Here's how the part is built. I have some questions about the finished solid (model axes, mm). Face numbers are marked on the shaded views. A direction names the side the tool comes from. Round coordinates to 2 decimals unless told otherwise and drop trailing zeros. Write each loop counter-clockwise with the first axis right and the second up, starting at its lowest first coordinate (ties: lowest second). Pieces come first, ordered by that corner, then holes. Notation, with made-up numbers: (2.25, -24.5) -> (18.25, -24.5) arc R14 ccw to (18.25, -5.5) -> close; hole circle Ø9 at (61.5, 24). An arc over 180 degrees is marked (long way). Put each result on its own line as item: value. Start each with the question number.
1) I want a section at B-B, the plane x = 23.5. List the corners of the cut face in (y, z) for me, then the cut area to 3 significant figures.
2) I want a section at C-C, the plane x = 7.5. List the corners of the cut face in (y, z) for me.
3) If I drill on line 1 along Z through (x, y) = (-34.5, -18.25); line 2 along Z through (x, y) = (38, -14); line 3 along Z through (x, y) = (35, -17), over which ranges is the centre line in solid material (lowest first)? Write a range as [from, to].
4) Will these pins go through, and if not, where does the flat tip stop? P1, Ø2, axis at y = -6, z = 25.5, coming from the -X side; P2, Ø1, axis at y = -19.5, z = 26.5, coming from the +X side; P3, Ø1, axis at x = 11, y = -19.5, coming from the +Z side.
5) Which directions (+Z, -Z, +X, -X, +Y, -Y) give clear straight access to the entire face, cutting with the end or side of a thin tool? Please do the marked faces 1 and 2.
6) I want a section at D-D, the plane z = 22.5. List the corners of the cut face in (x, y) for me, then the cut area to 3 significant figures.
7) I want a section at A-A, the plane y = -13.75. List the corners of the cut face in (x, z) for me.
from build123d import *

# Parameters (mm, degrees)
F1_DEPTH = 25


with BuildPart() as f1:
    # F0 (on Front) → F1 (new body)
    with BuildSketch(Plane.XZ):
        with BuildLine():
            Line((45.7854280798, 23.3870821038), (-39.147809339, 23.3870821038))
            ThreePointArc((-39.147809339, 23.3870821038), (-39.9978092392, 22.5370822037), (-39.147809339, 21.6870823036))
            Line((-39.147809339, 21.6870823036), (45.7854280798, 21.6870823036))
            ThreePointArc((45.7854280798, 21.6870823036), (46.0020177098, 21.6934270774), (46.2178645223, 21.7124396389))
            ThreePointArc((46.2178645223, 21.7124396389), (49.7941822228, 26.2093447117), (45.3231656181, 29.8179752068))
            Line((45.3231656181, 29.8179752068), (16.6060594099, 26.8574478911))
            ThreePointArc((16.6060594099, 26.8574478911), (16.2045950097, 26.8748577315), (15.8251544566, 27.0071514722))
            ThreePointArc((15.8251544566, 27.0071514722), (14.6830908852, 26.6449018554), (15.037802048, 25.5004744977))
            ThreePointArc((15.037802048, 25.5004744977), (15.8845244931, 25.2052607187), (16.7803932023, 25.1664106207))
            Line((16.7803932023, 25.1664106207), (45.4974994105, 28.1269379365))
            ThreePointArc((45.4974994105, 28.1269379365), (48.1044451468, 26.0228294719), (46.0191775208, 23.4007887723))
            ThreePointArc((46.0191775208, 23.4007887723), (45.9025035618, 23.3905117115), (45.7854280798, 23.3870821038))
        make_face()
    extrude(amount=F1_DEPTH)


solid = f1.part
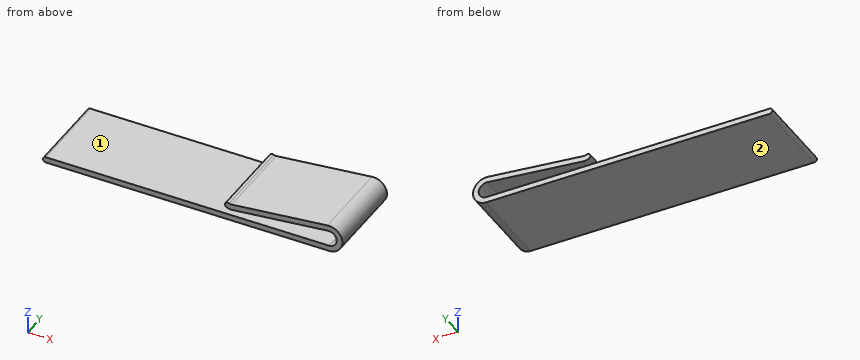
Findings:
1. outline: (-25, 21.69) -> (0, 21.69) -> (0, 23.39) -> (-25, 23.39) -> close; (-25, 25.86) -> (0, 25.86) -> (0, 27.57) -> (-25, 27.57) -> close
1. area: 85.2 mm2
2. outline: (-25, 21.69) -> (0, 21.69) -> (0, 23.39) -> (-25, 23.39) -> close
3. line 1: z = [21.69, 23.39]
3. line 2: z = [21.69, 23.39], [27.35, 29.06]
3. line 3: z = [21.69, 23.39], [27.04, 28.75]
4. P1: stops at x = 14.59
4. P2: stops at x = 49.81
4. P3: stops at z = 23.39
5. face 1: -X, +Y, -Y
5. face 2: -Z, +X, -X, +Y, -Y
6. outline: (-40, -25) -> (48.19, -25) -> (48.19, 0) -> (-40, 0) -> close
6. area: 2,200 mm2
7. outline: (-39.15, 21.69) -> (45.79, 21.69) arc R3.7 ccw to (46.22, 21.71) arc R4.08 ccw to (45.32, 29.82) -> (16.61, 26.86) arc R1.38 cw to (15.83, 27.01) arc R0.85 ccw to (15.04, 25.5) arc R3.08 ccw to (16.78, 25.17) -> (45.5, 28.13) arc R2.38 cw to (46.02, 23.4) arc R2 cw to (45.79, 23.39) -> (-39.15, 23.39) arc R0.85 ccw to start
